Geometry: final body of the model. Coordinates: model frame, mm. A direction names the side the tool comes from. Give positions to 0.01 mm unless a question says otherwise; leave off trailing zeros. Order: outer loops, then holes, each group sorted by start corner. A loop starts at its lowest first (then second) coordinate and runs counter-clockwise, first axis right, second up. Notation, with made-up numbers: (3.25, 53) -> (52.25, 53) arc R22 ccw to (52.25, 82) -> close; hole circle Ø8 at (55, 16). An arc over 180 degrees is marked (long way). Answer in a Markdown table with one row per item. Add a question column.
Q1. Pull-direction query (Z, two-part tool) for faces 1 (the face through (-30.895, 9.076, -0.242)), 2 (the face through (0, 25.4, 0)), 3 (the face through (-1, 10, 12.7)), 4 (the face through (-25, 5.35, 4)); classes: +Z half, -Z half, draft (parallel to the pull), parting line (faces both ways), or undercut.
Q2. Cut plane A-A on z = 0. Return the cut outline in (x, y), and give its area (3 significant figures).
Q3. Contact query for flat-ended pins moving along their axis: P1, Ø12, axis at x = -27.5, z = -6.5, coming from the +Y side; P2, Ø14, axis at y = 20.5, z = -5, coming from the +X side; P3, Ø1.5, axis at y = 13.5, z = -6.5, coming from the -X side. Output: stop coordinate, or through.
Q4. Cut plane D-D on z = 8.75. Return the cut outline in (x, y), and give its area (3 significant figures).
Q5. Line query: line 1 along X through (y, z) = (7, 0); line 2 along X through (y, z) = (2.95, 0); line 3 along Z through (x, y) = (25.4, 1.8). Output: solid intervals per line, ascending. Write a range as from..to.
Q6. Set-up query: faces 5 (the face through (25, 5.35, 4)), 6 (the face through (-12.7, 22, 3)), 7 (the face through (12.7, 22, 3)). Return all of +Z, -Z, +X, -X, +Y, -Y with unobstructed straight access to the full face (end or side cutting, diameter ignored); none if empty.
Q7. Cut plane B-B on y = 19.05. Return the cut outline in (x, z), and give its area (3 significant figures).
Q8. Cut plane C-C on x = -25.4. Return the cut outline in (y, z).
from build123d import *

# Parameters (mm, degrees)
SKETCH1_W           = 76.2
SKETCH1_H           = 25.4
SKETCH1_R           = 3.501199875
BOSS_EXTRUDE1_DEPTH = 12.7
SKETCH2_W           = 25.4
SKETCH2_H           = 25.4
BOSS_EXTRUDE2_DEPTH = 12.7
SKETCH3_R           = 4.001199875
CUT_EXTRUDE1_DEPTH  = 43.7
SKETCH4_R           = 5.5
CUT_EXTRUDE2_DEPTH  = 7.35


with BuildPart() as part:
    # Sketch1 → Boss-Extrude1 (new body)
    with BuildSketch(Plane(origin=(0, 0, 0), x_dir=(1, 0, 0), z_dir=(0, 1, 0))):
        Rectangle(SKETCH1_W, SKETCH1_H)
        with Locations((-25.4, 0)):
            Circle(SKETCH1_R, mode=Mode.SUBTRACT)
        with Locations((25.4, 0)):
            Circle(SKETCH1_R, mode=Mode.SUBTRACT)
    extrude(amount=BOSS_EXTRUDE1_DEPTH)

    # Sketch2 → Boss-Extrude2 (add)
    with BuildSketch(Plane(origin=(0, 12.7, 0), x_dir=(1, 0, 0), z_dir=(0, 1, 0))):
        Rectangle(SKETCH2_W, SKETCH2_H)
    extrude(amount=BOSS_EXTRUDE2_DEPTH)

    # Sketch3 → Cut-Extrude1 (cut)
    with BuildSketch(Plane.ZY.offset(12.7)):
        with Locations((0, 19.05)):
            Circle(SKETCH3_R)
    extrude(amount=-CUT_EXTRUDE1_DEPTH, mode=Mode.SUBTRACT)

    # Sketch4 → Cut-Extrude2 (cut)
    with BuildSketch(Plane(origin=(0, 12.7, 0), x_dir=(1, 0, 0), z_dir=(0, 1, 0))):
        with Locations((-25.4, 0)):
            Circle(SKETCH4_R)
        with Locations((25.4, 0)):
            Circle(SKETCH4_R)
    extrude(amount=-CUT_EXTRUDE2_DEPTH, mode=Mode.SUBTRACT)


solid = part.part
Completed:
| question | item | result |
|---|---|---|
| 1 | face 1 | undercut |
| 1 | face 2 | draft |
| 1 | face 3 | +Z half |
| 1 | face 4 | undercut |
| 2 | outline | (-38.1, 0) -> (-28.9, 0) -> (-28.9, 5.35) -> (-30.9, 5.35) -> (-30.9, 12.7) -> (-38.1, 12.7) -> close; (-21.9, 0) -> (21.9, 0) -> (21.9, 5.35) -> (19.9, 5.35) -> (19.9, 12.7) -> (12.7, 12.7) -> (12.7, 15.05) -> (-12.7, 15.05) -> (-12.7, 12.7) -> (-19.9, 12.7) -> (-19.9, 5.35) -> (-21.9, 5.35) -> close; (-12.7, 23.05) -> (12.7, 23.05) -> (12.7, 25.4) -> (-12.7, 25.4) -> close; (28.9, 0) -> (38.1, 0) -> (38.1, 12.7) -> (30.9, 12.7) -> (30.9, 5.35) -> (28.9, 5.35) -> close |
| 2 | area | 850 mm² |
| 3 | P1 | stops at y = 12.7 |
| 3 | P2 | stops at x = 12.7 |
| 3 | P3 | stops at x = -12.7 |
| 4 | outline | (-38.1, 0) -> (38.1, 0) -> (38.1, 12.7) -> (12.7, 12.7) -> (12.7, 25.4) -> (-12.7, 25.4) -> (-12.7, 12.7) -> (-38.1, 12.7) -> close |
| 4 | area | 1,290 mm² |
| 5 | line 1 | x = -38.1..-30.9, -19.9..19.9, 30.9..38.1 |
| 5 | line 2 | x = -38.1..-28.9, -21.9..21.9, 28.9..38.1 |
| 5 | line 3 | z = -12.7..-3.5, 3.5..12.7 |
| 6 | face 5 | +Y |
| 6 | face 6 | +Z, -Z, -X, +Y |
| 6 | face 7 | +Z, -Z, +X, +Y |
| 7 | outline | (-12.7, -12.7) -> (12.7, -12.7) -> (12.7, -4) -> (-12.7, -4) -> close; (-12.7, 4) -> (12.7, 4) -> (12.7, 12.7) -> (-12.7, 12.7) -> close |
| 7 | area | 442 mm² |
| 8 | outline | (0, -12.7) -> (12.7, -12.7) -> (12.7, -5.5) -> (5.35, -5.5) -> (5.35, -3.5) -> (0, -3.5) -> close; (0, 3.5) -> (5.35, 3.5) -> (5.35, 5.5) -> (12.7, 5.5) -> (12.7, 12.7) -> (0, 12.7) -> close |
